from build123d import *

# Parameters (mm, degrees)
F0_W     = 1315
F0_H     = 1350
F1_DEPTH = 100
F2_W     = 1100
F2_H     = 1135
F3_DEPTH = 30


with BuildPart() as f1:
    # F0 (on Top) → F1 (new body)
    with BuildSketch(Plane.XY):
        Rectangle(F0_W, F0_H)
    extrude(amount=F1_DEPTH)

    # F2 (on face) → F3 (cut)
    with BuildSketch(Plane.XY.offset(100)):
        Rectangle(F2_W, F2_H)
    extrude(amount=-F3_DEPTH, mode=Mode.SUBTRACT)

    # F6: sweep along a path in F5
    with BuildLine(Plane.XY.offset(70)) as f6_path:
        Line((550, 567.5), (550, -567.5))
        Line((550, -567.5), (-550, -567.5))
        Line((-550, -567.5), (-550, 567.5))
        Line((-550, 567.5), (550, 567.5))
    # F4 (on Right) → F6 (sweep)
    with BuildSketch(Plane.YZ):
        with BuildLine():
            Line((-567.5, 100), (-567.5, 70))
            Line((-567.5, 70), (-532.1858882904, 70))
            Line((-532.1858882904, 70), (-532.1858882904, 75))
            ThreePointArc((-532.1858882904, 75), (-546.3280239141, 80.8578643763), (-552.1858882904, 95))
            Line((-552.1858882904, 95), (-557.1858882904, 95))
            Line((-557.1858882904, 95), (-557.1858882904, 100))
            Line((-557.1858882904, 100), (-567.5, 100))
        make_face()
    sweep(path=f6_path.line, transition=Transition.RIGHT)


solid = f1.part
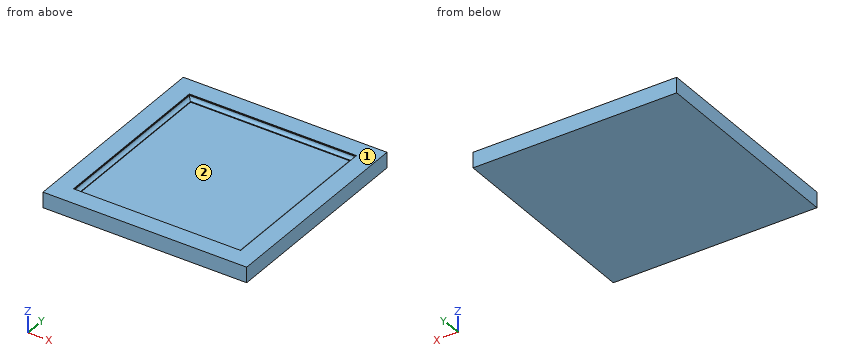
Design review of the part built by this model. Coordinates are the model's own, in mm. Face numbers are marked on the shaded views. Round coordinates to 2 decimals unless told otherwise and drop trailing zeros. Order: outer loops, then holes, each group sorted by start corner. A loop starts at its lowest first (then second) coordinate and runs counter-clockwise, first axis right, second up.
1) Consider section A-A (y = 101.5). State the section outline as (x, z) points.
The answers:
outline: (-657.5, 0) - (657.5, 0) - (657.5, 100) - (539.69, 100) - (539.69, 95) - (534.69, 95) arc R20 cw to (514.69, 75) - (514.69, 70) - (-514.69, 70) - (-514.69, 75) arc R20 cw to (-534.69, 95) - (-539.69, 95) - (-539.69, 100) - (-657.5, 100) - close
2) For L1, parallel to X at y = 266.5, z = 70.5; L2, parallel to X at y = 457.5, z = 92; L3, parallel to Z at x = 311, y = 119, list the stretches that pass through material, from the lowest coordinate up.
The answers:
L1: x = -657.5 to -514.69, 514.69 to 657.5
L2: x = -657.5 to -534.46, 534.46 to 657.5
L3: z = 0 to 70
3) Consider section B-B (x = -255). State the section outline as (y, z) points, plus the area to 3 significant figures.
The answers:
outline: (-675, 0) - (675, 0) - (675, 100) - (557.19, 100) - (557.19, 95) - (552.19, 95) arc R20 cw to (532.19, 75) - (532.19, 70) - (-532.19, 70) - (-532.19, 75) arc R20 cw to (-552.19, 95) - (-557.19, 95) - (-557.19, 100) - (-675, 100) - close
area: 102,000 mm2
4) Clearance check with a flat-ended pin moving along its axis: pin 1 Ø2 at (x, y) = (-77, 331) entering from +Z. State where the tip first meets the part, or that it passes through.
The answers:
pin 1: stops at z = 70
5) Draft analysis for pull direction Y (two halves, no side actions). For the marked faces 1 and 2, state which applies: released by +Y, released by -Y, zero draft, split by the parting line, or undercut.
The answers:
face 1: zero draft
face 2: undercut
